Geometry check sheet. Reference: the model listing, model coordinates, mm. Face numbers are marked on the shaded views. A direction names the side the tool comes from. Coordinates: 2 decimals unless noted, no trailing zeros. Write each loop counter-clockwise with the first axis right and the second up, starting at its lowest first coordinate (ties: lowest second). Pieces come first, ordered by that corner, then holes. Notation, with made-up numbers: (-24.5, 34.5) -> (24.5, 34.5) arc R16 ccw to (24.5, 56.5) -> close; hole circle Ø1 at (23.25, 10). An arc over 180 degrees is marked (long way). One line per question, with ' | ' between items.
from build123d import *

# Parameters (mm, degrees)
SKETCH2_R                     = 6.35
SKETCH4_R                     = 6.35
COLUMN_DEPTH                  = 12.7
SKETCH5_R                     = 3.175
FASTENER_HOLE_CUT_DEPTH       = 42.503942147
COLUMN_AND_HOLE_PATTERN_COUNT = 4


with BuildPart() as part:
    # Sketch2 → Base Revolve (revolve)
    with BuildSketch(Plane.XY, mode=Mode.PRIVATE) as base_revolve_sk:
        with Locations((21.59, 0)):
            Circle(SKETCH2_R)
    revolve(base_revolve_sk.sketch.rotate(Axis((0, 0, 0), (0, 1, 0)), 90), axis=Axis((0, 0, 0), (0, 1, 0)))

    # Sketch4 → Column (add, symmetric)
    with BuildSketch(Plane(origin=(0, 0, 0), x_dir=(1, 0, 0), z_dir=(0, 1, 0))):
        with Locations(Location((0, 21.59, 0), (0, 0, 270))):
            Circle(SKETCH4_R)
    column = extrude(amount=COLUMN_DEPTH, both=True)

    # Sketch5 → Fastener Hole Cut (cut, symmetric)
    with BuildSketch(Plane(origin=(0, 0, 0), x_dir=(1, 0, 0), z_dir=(0, 1, 0))):
        with Locations(Location((0, 21.59, 0), (0, 0, 270))):
            Circle(SKETCH5_R)
    fastener_hole_cut = extrude(amount=FASTENER_HOLE_CUT_DEPTH, both=True, mode=Mode.SUBTRACT)

    # Column and Hole Pattern: Column, Fastener Hole Cut ×4 about axis
    column_and_hole_pattern_axis = Axis((0, 0, 0), (0, 1, 0))
    add([column.rotate(column_and_hole_pattern_axis, i * 360 / COLUMN_AND_HOLE_PATTERN_COUNT) for i in range(1, COLUMN_AND_HOLE_PATTERN_COUNT)])
    add([fastener_hole_cut.rotate(column_and_hole_pattern_axis, i * 360 / COLUMN_AND_HOLE_PATTERN_COUNT) for i in range(1, COLUMN_AND_HOLE_PATTERN_COUNT)], mode=Mode.SUBTRACT)


solid = part.part
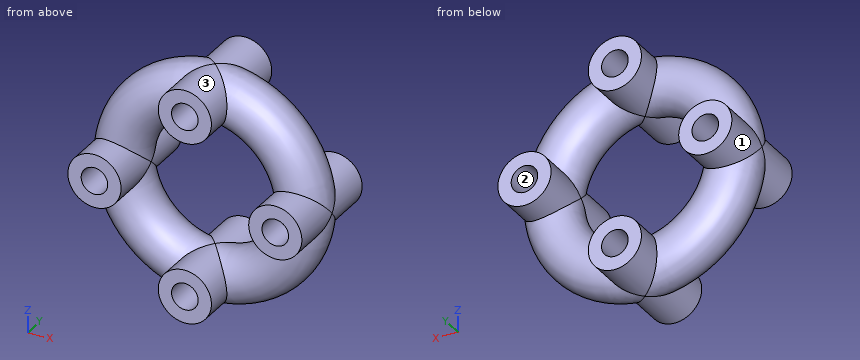
1. Go/stop test with flat-tipped pins: P1, Ø2, axis at y = -4.5, z = 22, coming from the +X side; P2, Ø1, axis at x = -18.5, z = -16.5, coming from the -Y side; P3, Ø1.5, axis at x = -4.5, y = -5.5, coming from the +Z side. Record where each tip stops, or that it passes through.
Worked answers:
P1: x = 16.08 | P2: y = -5.75 | P3: z = 26.71
2. Cross-section at B-B on y = 1.25. Give the number of separate pieces and of enclosed holes in the cut face, and give its area (3 significant figures).
Worked answers:
separate pieces: 1 | enclosed holes: 5 | area: 1,560 mm²
3. Cross-section at A-A on y = 11.25. Record the boundary of the cut face in (x, z) (3 decimals).
Worked answers:
outline: circle Ø12.7 at (-21.59, 0); circle Ø12.7 at (0, -21.59); circle Ø12.7 at (0, 21.59); circle Ø12.7 at (21.59, 0); hole circle Ø6.35 at (-21.59, 0); hole circle Ø6.35 at (0, -21.59); hole circle Ø6.35 at (0, 21.59); hole circle Ø6.35 at (21.59, 0)
4. Tool access check on the marked faces 1, 2 and 3. Record the directions out of +Z, -Z, +X, -X, +Y, -Y that give a thin tool (end or side, any length) a straight path to the whole face; none if there is none.
Worked answers:
face 1: +Y | face 2: +Y, -Y | face 3: -Y
5. Material ranges on line 1 (X direction, y = -7.5, z = 21.59) (3 decimals); line 2 (X direction, y = -1.75, z = -2); line 3 (Y direction, x = -19, z = 11), recorded low to high. Write a range as from..to.
Worked answers:
line 1: -6.35..-3.175, 3.175..6.35 | line 2: -27.62..-24.06, -19.12..-15.36, 15.36..19.12, 24.06..27.62 | line 3: -6.34..6.34
